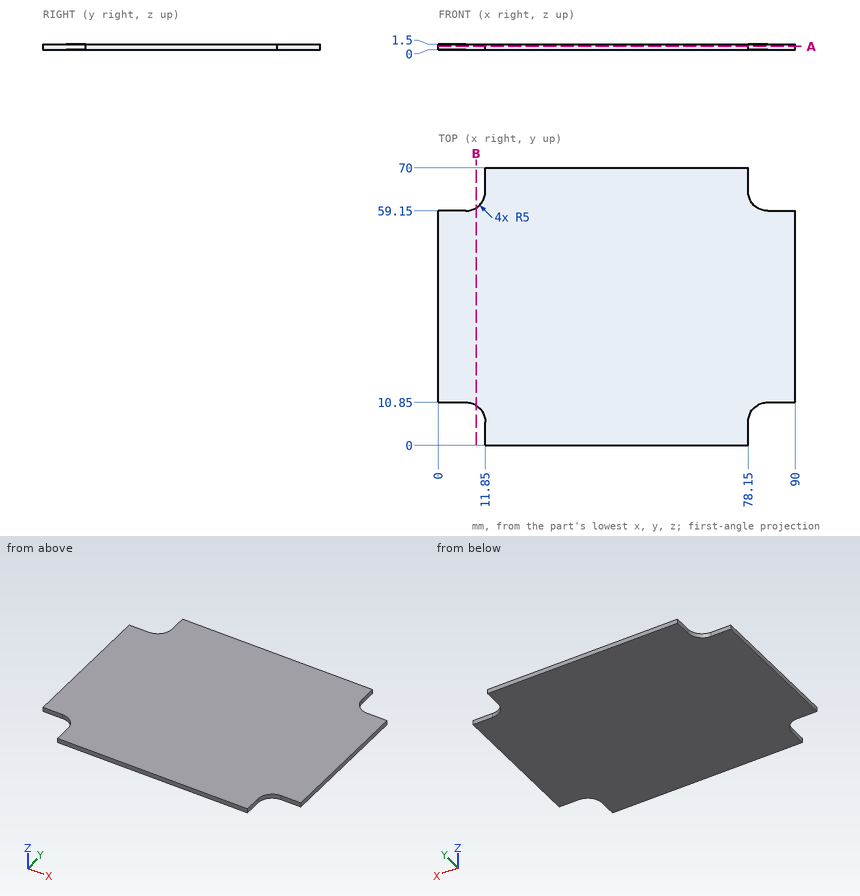
Study the drawing (mm; zero at the part's minimum x, y, z) and answer. Give positions to 0.01 mm unless a question says otherwise; leave off trailing zeros. Write each loop counter-clockwise with the first axis right and the second up, starting at its lowest first coordinate (ties: lowest second). Pieces come first, ordered by that corner, then holes. Notation, with made-up numbers: (-39, 52) -> (18, 52) arc R4 ccw to (18, 56) -> close; hole circle Ø7 at (55.25, 4.25). An arc over 180 degrees is marked (long way). Answer as a JSON object with one key per item and string values. Group by question number.
1) Find section A-A (z = 0.9). Write down the section's boundary in (x, y), and give its area (3 significant figures).
2) Each of these flat-tipped pins is pushed along its axis until it touches: P1, Ø0.8, axis at x = 2, z = 1, coming from the +Y side; P2, Ø0.8, axis at x = 4, z = 0.5, coming from the -Y side. Where does it stop, or does it pass through?
3) Find section B-B (x = 9.5). Write down the section's boundary in (y, z), and give its area (3 significant figures).
4) Consider L1, parallel to X at y = 3.5, z = 1; L2, parallel to Y at x = 6.5, z = 1. Determine where each line is inside the solid, lowest interval first. Write a range as from..to.
Values follow:
{
 "1": {"outline": "(0, 10.85) -> (6.85, 10.85) arc R5 cw to (11.85, 5.85) -> (11.85, 0) -> (78.15, 0) -> (78.15, 5.85) arc R5 cw to (83.15, 10.85) -> (90, 10.85) -> (90, 59.15) -> (83.15, 59.15) arc R5 cw to (78.15, 64.15) -> (78.15, 70) -> (11.85, 70) -> (11.85, 64.15) arc R5 cw to (6.85, 59.15) -> (0, 59.15) -> close", "area": "5,810 mm2"},
 "2": {"P1": "stops at y = 59.15", "P2": "stops at y = 10.85"},
 "3": {"outline": "(10.09, 0) -> (59.91, 0) -> (59.91, 1.5) -> (10.09, 1.5) -> close", "area": "74.7 mm2"},
 "4": {"L1": "x = 11.85..78.15", "L2": "y = 10.85..59.15"}
}
